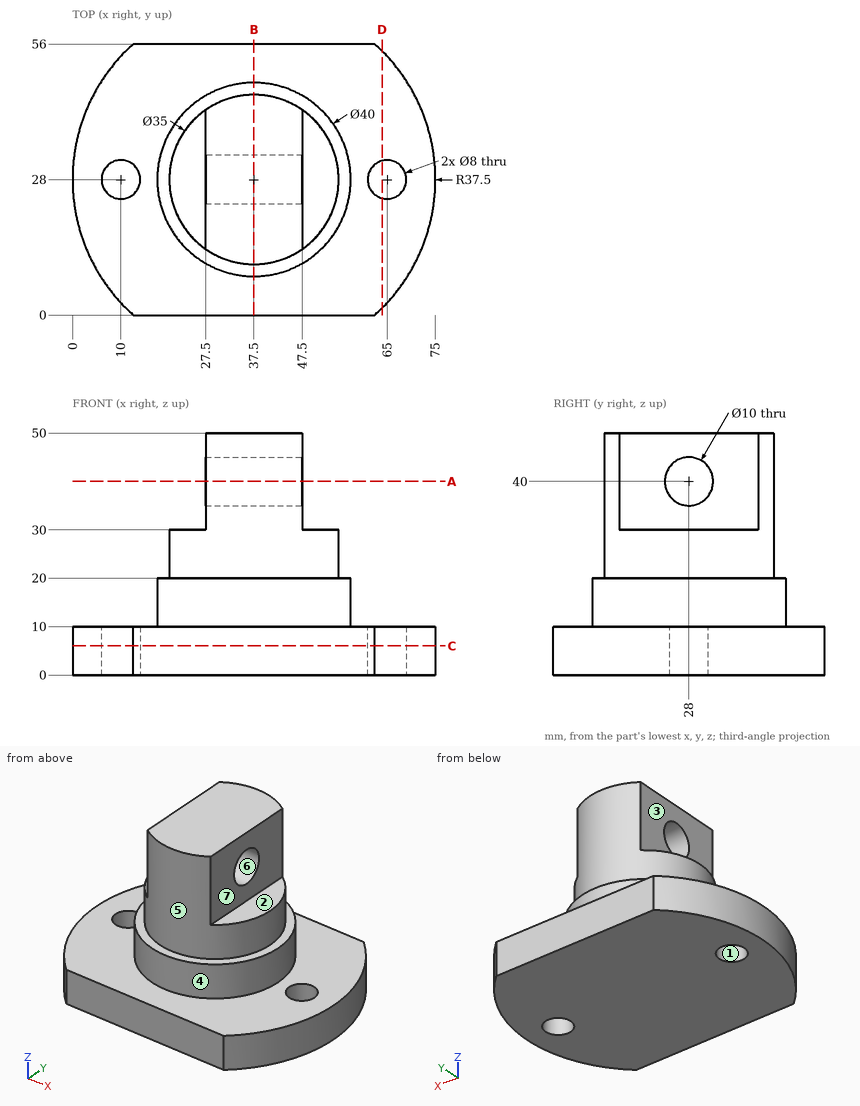
Job drawing, mm, ordinate dimensions from the low corner. One solid piece. A direction names the side the tool comes from. Give positions to 0.01 mm unless a question says otherwise; leave off trailing zeros. Loops run counter-clockwise (first coordinate to the right, second up) from the corner with the lowest first, then second, coordinate; pieces in that order, holes last. Notation, with made-up numbers: (-28.5, -35.75) - (29.5, -35.75) arc R31 ccw to (29.5, -8.75) - close; hole circle Ø4 at (-33.75, 17). An arc over 180 degrees is marked (long way). Use one line per item in the form item = value.
(1) 3-axis set-ups, long thin cutter, end or side, ignore diameter. For the marked faces 1, 2, 3 and 4: which of +Z, -Z, +X, -X, +Y, -Y reach the whole face in a straight line?
Determined:
face_1 = +Z, -Z
face_2 = +Z, +X, +Y, -Y
face_3 = +Z, -X, +Y, -Y
face_4 = +Z
(2) Cut at A-A (z = 40). Give the cut face in (x, y), then the cut area to 3 significant figures.
Determined:
outline = (27.5, 13.64) arc R17.5 ccw to (47.5, 13.64) - (47.5, 23) - (27.5, 23) - close; (27.5, 33) - (47.5, 33) - (47.5, 42.36) arc R17.5 ccw to (27.5, 42.36) - close
area = 460 mm^2
(3) Cut at D-D (x = 64). Give the cut face in (y, z), then the cut area to 3 significant figures.
Determined:
outline = (1.47, 0) - (24.13, 0) - (24.13, 10) - (1.47, 10) - close; (31.87, 0) - (54.53, 0) - (54.53, 10) - (31.87, 10) - close
area = 453 mm^2
(4) Pull direction Y, two halves, no side cores. Call the marked faces 5, 6 and 7: pulls with the +Y half, pulls with the -Y half, needs draft (parallel to the pull), parting line crosses it, or undercut.
Determined:
face_5 = parting line crosses it
face_6 = undercut
face_7 = needs draft
(5) Cut at B-B (x = 37.5). Give the cut face in (y, z).
Determined:
outline = (0, 0) - (56, 0) - (56, 10) - (48, 10) - (48, 20) - (45.5, 20) - (45.5, 50) - (10.5, 50) - (10.5, 20) - (8, 20) - (8, 10) - (0, 10) - close; hole circle Ø10 at (28, 40)
(6) Drill centre lines: L1, parallel to X at y = 33, z = 42; L2, parallel to Z at x = 19.5, y = 31; L3, parallel to Z at x = 34.5, y = 28. Where is each one in solid material? Low to high.
Determined:
L1 = 27.5 to 47.5
L2 = 0 to 20
L3 = 0 to 35, 45 to 50
(7) Cut at C-C (z = 6). Give the cut face in (x, y).
Determined:
outline = (12.56, 0) - (62.44, 0) arc R37.5 ccw to (62.44, 56) - (12.56, 56) arc R37.5 ccw to start; hole circle Ø8 at (10, 28); hole circle Ø8 at (65, 28)
(8) Drop flat-ended pins along their axis: P1, Ø9, axis at y = 28, z = 40, coming from the -X side; P2, Ø2, axis at y = 29.5, z = 27.5, coming from the -X side; P3, Ø6, axis at y = 26.5, z = 37.5, coming from the +X side; P4, Ø5, axis at x = 28.5, z = 20.5, coming from the +Y side. Give the stop position or say it passes through.
Determined:
P1 = through
P2 = 20.01
P3 = 47.5
P4 = 46.9
